Answer from the drawing. Dimensions are ordinates in mm from the lowest x, y and z of the part. Coordinates: 2 decimals unless noted, no trailing zeros. Loops run counter-clockwise (first coordinate to the right, second up) from the corner with the lowest first, then second, coordinate; pieces in that order, holes last. Notation, with made-up numbers: M 4.25,42.5 L 22.25,42.5 A11 ccw 22.25,61.5 Z; hole C -34,54.25 d4. An arc over 180 degrees is marked long. Put each result on its own line as item: value.
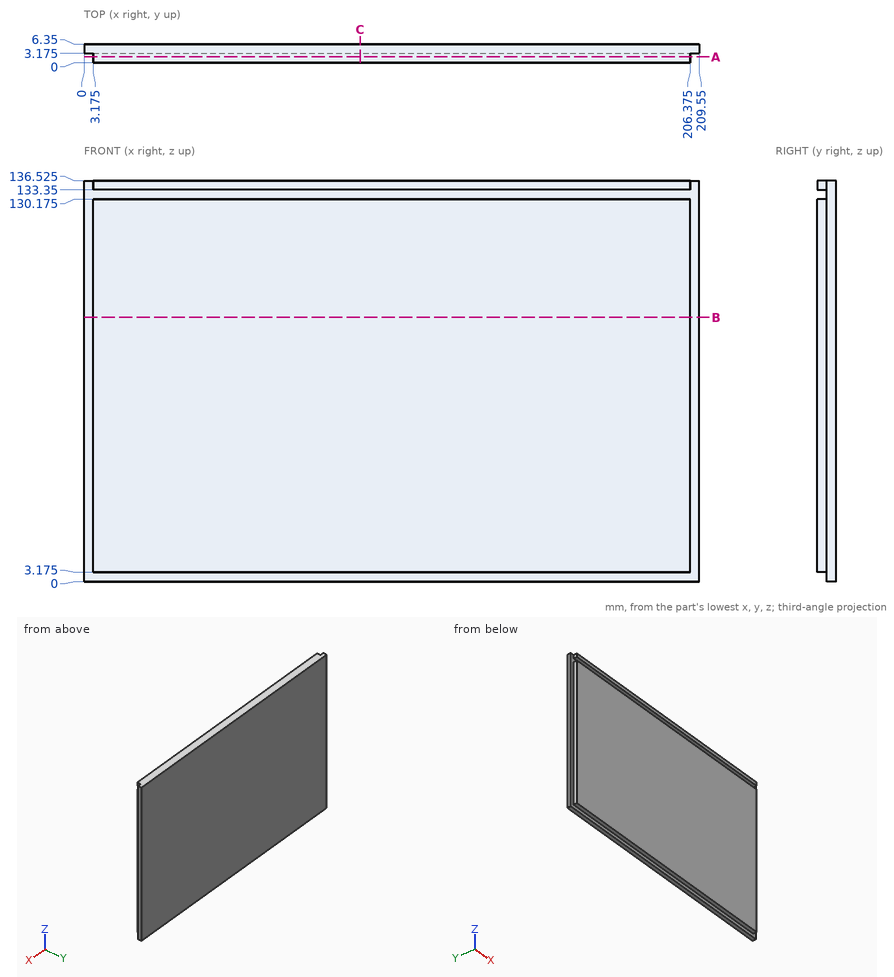
1) Find section A-A, the plane y = 2. Write down the section's boundary in (x, z) (3 decimals), plus the area to 3 significant figures.
Answer list:
outline: M 3.175,3.175 L 206.375,3.175 L 206.375,130.175 L 3.175,130.175 Z; M 3.175,133.35 L 206.375,133.35 L 206.375,136.525 L 3.175,136.525 Z
area: 26,500 mm^2
2) Straight lines are drawn through the part: line 1 (Z direction, x = 15, y = 1) (3 decimals); line 2 (X direction, y = 2.75, z = 75) (3 decimals). For each, find the intervals that lie inside material, in ascending order. Write a range as [from, to].
Answer list:
line 1: z = [3.175, 130.175], [133.35, 136.525]
line 2: x = [3.175, 206.375]
3) Find section C-C, the plane x = 94. Write down the section's boundary in (y, z) (3 decimals), plus the area to 3 significant figures.
Answer list:
outline: M 0,3.175 L 3.175,3.175 L 3.175,0 L 6.35,0 L 6.35,136.525 L 0,136.525 L 0,133.35 L 3.175,133.35 L 3.175,130.175 L 0,130.175 Z
area: 847 mm^2
4) Find section B-B, the plane z = 90. Write down the section's boundary in (x, y) (3 decimals).
Answer list:
outline: M 0,3.175 L 3.175,3.175 L 3.175,0 L 206.375,0 L 206.375,3.175 L 209.55,3.175 L 209.55,6.35 L 0,6.35 Z
5) Given pin 1 Ø1 at (y, z) = (1.5, 59) entering from +X (3 decimals); pin 2 Ø1 at (x, y) = (77.5, 2) entering from -Z (3 decimals); pin 3 Ø1.6 at (y, z) = (1.5, 64.5) entering from -X (3 decimals), each flat-ended and moving along its own axis, determine where each tip first touches the part or whether it passes through.
Answer list:
pin 1: stops at x = 206.375
pin 2: stops at z = 3.175
pin 3: stops at x = 3.175
